Could you check a few things on this model? Use its own coordinates, in mm. Round coordinates to 2 decimals unless told otherwise and drop trailing zeros. Loops run counter-clockwise (first coordinate to the right, second up) from the corner with the lowest first, then second, coordinate; pieces in that order, holes last.
from build123d import *

# Parameters (mm, degrees)
SKETCH1_W           = 10
SKETCH1_H           = 10
BOSS_EXTRUDE1_DEPTH = 150
SKETCH2_R           = 2.5
BOSS_EXTRUDE2_DEPTH = 3
SKETCH3_R           = 1.25
BOSS_EXTRUDE3_DEPTH = 6


with BuildPart() as part:
    # Sketch1 → Boss-Extrude1 (new body)
    with BuildSketch(Plane.XY):
        with Locations((5, -5)):
            Rectangle(SKETCH1_W, SKETCH1_H)
    extrude(amount=BOSS_EXTRUDE1_DEPTH)

    # Sketch2 → Boss-Extrude2 (add)
    with BuildSketch(Plane.XZ.offset(10)):
        with Locations(Location((5, 145, 0), (0, 0, 90))):
            Circle(SKETCH2_R)
    extrude(amount=BOSS_EXTRUDE2_DEPTH)

    # Sketch3 → Boss-Extrude3 (add)
    with BuildSketch(Plane.XZ.offset(10)):
        with Locations(Location((5, 145, 0), (0, 0, 270))):
            Circle(SKETCH3_R)
    extrude(amount=BOSS_EXTRUDE3_DEPTH)


solid = part.part
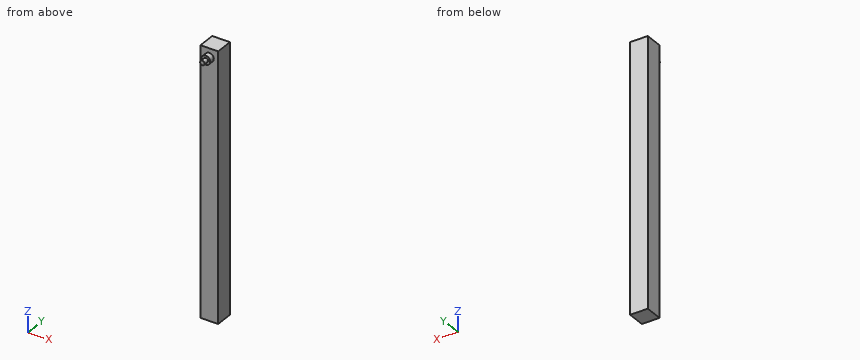
Item 1: If I drill on line 1 along Y through (x, z) = (6.5, 94); line 2 along Z through (x, y) = (5.25, -11.75); line 3 along Z through (x, y) = (7.25, -11.25), over which ranges is the centre line in solid material (lowest first)?
Results list:
line 1: y = -10 to 0
line 2: z = 142.51 to 147.49
line 3: z = 143.91 to 146.09
Item 2: Will this pin go through, and if not, where does the flat tip stop? pin 1 (5 mm diameter, centred on x = 7, z = 111, fed in from -Y).
Results list:
pin 1: stops at y = -10
Item 3: If we section it at D-D, the plane z = 126: Please give me the cut outline in (x, y).
Results list:
outline: (0, -10) - (10, -10) - (10, 0) - (0, 0) - close
Item 4: If we section it at B-B, the plane x = 5: Please give me the cut outline in (y, z).
Results list:
outline: (-16, 143.75) - (-13, 143.75) - (-13, 142.5) - (-10, 142.5) - (-10, 0) - (0, 0) - (0, 150) - (-10, 150) - (-10, 147.5) - (-13, 147.5) - (-13, 146.25) - (-16, 146.25) - close
Item 5: If we section it at C-C, the plane y = -11.75: Please give me the cut outline in (x, z), then the cut area to 3 significant figures.
Results list:
outline: circle Ø5 at (5, 145)
area: 19.6 mm2
Item 6: If we section it at A-A, the plane z = 145: Please give me the cut outline in (x, y), then the cut area to 4 significant figures.
Results list:
outline: (0, -10) - (2.5, -10) - (2.5, -13) - (3.75, -13) - (3.75, -16) - (6.25, -16) - (6.25, -13) - (7.5, -13) - (7.5, -10) - (10, -10) - (10, 0) - (0, 0) - close
area: 122.5 mm2
